```python
from build123d import *

# Parameters (mm, degrees)
BOSS_EXTRUDE1_DEPTH = 1.5875
SKETCH2_W           = 4.5
SKETCH2_H           = 3.5
CUT_EXTRUDE1_DEPTH  = 2.5875
CHAMFER1_SIZE       = 1
SKETCH3_W           = 7.62
SKETCH3_H           = 7.62
BOSS_EXTRUDE2_DEPTH = 2.9718
FILLET1_R           = 0.508


with BuildPart() as part:
    # Sketch1 → Boss-Extrude1 (new body)
    with BuildSketch(Plane.XY):
        with BuildLine():
            Line((4.207, 4.461), (-4.207, 4.461))
            ThreePointArc((-4.207, 4.461), (-4.386605122, 4.386605122), (-4.461, 4.207))
            Line((-4.461, 4.207), (-4.461, -4.207))
            ThreePointArc((-4.461, -4.207), (-4.386605122, -4.386605122), (-4.207, -4.461))
            Line((-4.207, -4.461), (4.207, -4.461))
            ThreePointArc((4.207, -4.461), (4.386605122, -4.386605122), (4.461, -4.207))
            Line((4.461, -4.207), (4.461, 4.207))
            ThreePointArc((4.461, 4.207), (4.386605122, 4.386605122), (4.207, 4.461))
        make_face()
    extrude(amount=BOSS_EXTRUDE1_DEPTH)

    # Sketch2 → Cut-Extrude1 (cut, through all)
    with BuildSketch(Plane.XY.offset(1.5875)):
        Rectangle(SKETCH2_W, SKETCH2_H)
    extrude(amount=-CUT_EXTRUDE1_DEPTH, mode=Mode.SUBTRACT)

    # Chamfer1
    chamfer1_edges = [part.edges().sort_by_distance(p)[0] for p in [
        (2.25, 1.75, 0.79375),
        (2.25, -1.75, 0.79375),
        (-2.25, -1.75, 0.79375),
        (-2.25, 1.75, 0.79375),
    ]]
    chamfer(chamfer1_edges, length=CHAMFER1_SIZE)

    # Sketch3 → Boss-Extrude2 (add)
    with BuildSketch(Plane(origin=(0, 0, 0), x_dir=(-1, 0, 0), z_dir=(0, 0, -1))):
        Rectangle(SKETCH3_W, SKETCH3_H)
        Polygon((2.25, -0.75), (2.25, 0.75), (1.25, 1.75), (-1.25, 1.75), (-2.25, 0.75), (-2.25, -0.75), (-1.25, -1.75), (1.25, -1.75), align=None, mode=Mode.SUBTRACT)
    extrude(amount=BOSS_EXTRUDE2_DEPTH)

    # Fillet1
    fillet1_edges = [part.edges().sort_by_distance(p)[0] for p in [
        (3.81, 3.81, -1.4859),
        (3.81, -3.81, -1.4859),
        (-3.81, -3.81, -1.4859),
        (-3.81, 3.81, -1.4859),
    ]]
    fillet(fillet1_edges, radius=FILLET1_R)


solid = part.part
```
CAD build for the part. Positions are in the model's coordinates, mm. A direction names the side the tool comes from. Coordinates: 2 decimals unless noted, no trailing zeros. Write each loop counter-clockwise with the first axis right and the second up, starting at its lowest first coordinate (ties: lowest second). Pieces come first, ordered by that corner, then holes. Notation, with made-up numbers: (27, -36) -> (75, -36) arc R6 ccw to (75, -31) -> close; hole circle Ø9 at (63, 65.5). An arc over 180 degrees is marked (long way). Return JSON: item names as keys, results as strings. Group by question number.
Q1. Cut at C-C, the plane x = 0.25. Give the cut face in (y, z).
Q2. Which spindle directions (+Z, -Z, +X, -X, +Y, -Y) get a long thin tool onto all of the face, cutting with end or side? Do faces 4 (the face through (0, -3.81, -1)), 5 (the face through (-2.25, 0, -1)), 6 (the face through (-4, 0, 0)). Say none if no direction does.
Q3. Cut at D-D, the plane y = 3. Give the cut face in (x, z).
Q4. Cut at A-A, the plane y = -0.5. Give the cut face in (x, z), then the cut area to 3 significant figures.
Q5. Pull direction Y, two halves, no side cores. Call faces 1 (the face through (0, 3.81, -1)), 2 (the face through (4.461, 0, 1)), 3 (the face through (-2, -1, -1)): released by +Y, released by -Y, zero draft, split by the parting line, or undercut.
Q6. Drill centre lines: line 1 (Y direction, x = -0.75, z = -0.2); line 2 (X direction, y = 0.5, z = -0.85); line 3 (Y direction, x = 1.75, z = 0.1). Where is each one in solid material? Low to high.
Q7. Cut at B-B, the plane z = -1.95. Give the cut face in (x, y), then the cut area to 3 significant figures.
Q8. Flat gauge pins, fed straight in: pin 1 (1.5 mm diameter, centred on x = -1.5, z = -1, fed in from -Y); pin 2 (4.5 mm diameter, centred on x = 0, y = -1.5, fed in from -Z); pin 3 (1.5 mm diameter, centred on y = 0, z = -1.5, fed in from -X); pin 4 (1.2 mm diameter, centred on x = 0, z = -1, fed in from +Y). Where does each tip first touch, or does it go through?
Returned:
{
 "1": {"outline": "(-4.46, 0) -> (-3.81, 0) -> (-3.81, -2.97) -> (-1.75, -2.97) -> (-1.75, 1.59) -> (-4.46, 1.59) -> close; (1.75, -2.97) -> (3.81, -2.97) -> (3.81, 0) -> (4.46, 0) -> (4.46, 1.59) -> (1.75, 1.59) -> close"},
 "2": {"face 4": "-Z, +X, -X, -Y", "face 5": "+Z, -Z", "face 6": "-Z"},
 "3": {"outline": "(-4.46, 0) -> (-3.81, 0) -> (-3.81, -2.97) -> (3.81, -2.97) -> (3.81, 0) -> (4.46, 0) -> (4.46, 1.59) -> (-4.46, 1.59) -> close"},
 "4": {"outline": "(-4.46, 0) -> (-3.81, 0) -> (-3.81, -2.97) -> (-2.25, -2.97) -> (-2.25, 1.59) -> (-4.46, 1.59) -> close; (2.25, -2.97) -> (3.81, -2.97) -> (3.81, 0) -> (4.46, 0) -> (4.46, 1.59) -> (2.25, 1.59) -> close", "area": "16.3 mm2"},
 "5": {"face 1": "released by +Y", "face 2": "zero draft", "face 3": "undercut"},
 "6": {"line 1": "y = -3.81 to -1.75, 1.75 to 3.81", "line 2": "x = -3.81 to -2.25, 2.25 to 3.81", "line 3": "y = -4.46 to -1.25, 1.25 to 4.46"},
 "7": {"outline": "(-3.81, -3.3) arc R0.51 ccw to (-3.3, -3.81) -> (3.3, -3.81) arc R0.51 ccw to (3.81, -3.3) -> (3.81, 3.3) arc R0.51 ccw to (3.3, 3.81) -> (-3.3, 3.81) arc R0.51 ccw to (-3.81, 3.3) -> close; hole (-2.25, -0.75) -> (-1.25, -1.75) -> (1.25, -1.75) -> (2.25, -0.75) -> (2.25, 0.75) -> (1.25, 1.75) -> (-1.25, 1.75) -> (-2.25, 0.75) -> close", "area": "44.1 mm2"},
 "8": {"pin 1": "stops at y = -3.81", "pin 2": "stops at z = -2.97", "pin 3": "stops at x = -3.81", "pin 4": "stops at y = 3.81"}
}
